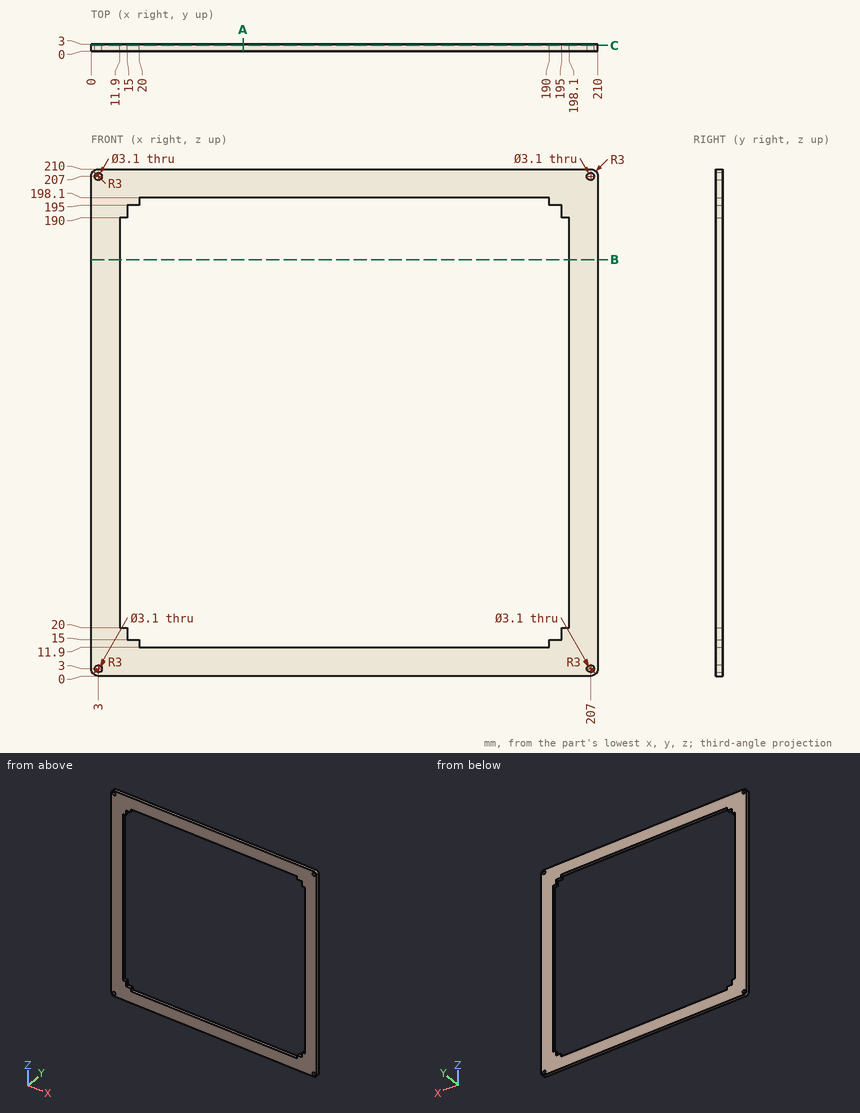
Check sheet for the drawn part. Datum: minimum x, y, z corner. Units: mm. Give positions to 0.01 mm unless a question says otherwise; leave off trailing zeros. Write each loop counter-clockwise with the first axis right and the second up, starting at its lowest first coordinate (ties: lowest second). Pieces come first, ordered by that corner, then holes.
(1) Cross-section at B-B (z = 172.5). Enter the section's corners in (x, y), plus the area to 3 significant figures.
(2) Cross-section at C-C (y = 2.45). State how many separate pieces and enclosed holes the cut face has, plus the area to 3 significant figures.
(3) Gauge pin test, flat end, axial feed: pin 1 (4 mm diameter, centred on x = 207, z = 3, fed in from -Y). Record the tip position at first contact, or that the pin passes through.
(4) Cross-section at A-A (x = 63). Enter the section's corners in (y, z).
(5) Material ranges on line 1 (X direction, y = 2.4, z = 207); line 2 (Z direction, x = 68.5, y = 2.2), recorded low to high.
Worked out:
1. outline: (0, 0) - (11.9, 0) - (11.9, 3) - (0, 3) - close; (198.1, 0) - (210, 0) - (210, 3) - (198.1, 3) - close
1. area: 71.4 mm2
2. separate pieces: 1
2. enclosed holes: 5
2. area: 9,550 mm2
3. pin 1: stops at y = 0
4. outline: (0, 0) - (3, 0) - (3, 11.9) - (0, 11.9) - close; (0, 198.1) - (3, 198.1) - (3, 210) - (0, 210) - close
5. line 1: x = 0 to 1.45, 4.55 to 205.45, 208.55 to 210
5. line 2: z = 0 to 11.9, 198.1 to 210
